Here's the drawing with two shaded views (mm, measured from the low corner). I have some questions. A direction names the side the tool comes from. Give positions to 0.01 mm unless a question says otherwise; leave off trailing zeros. Loops run counter-clockwise (first coordinate to the right, second up) from the corner with the lowest first, then second, coordinate; pieces in that order, holes last. Notation, with made-up numbers: M 4,33.5 L 30,33.5 A26 cw 30,52.5 Z; hole C -34,10 d8. An arc over 180 degrees is marked long. Use a Markdown table: item, result. Add a question column.
1) Suppose I cut it at D-D on x = 24. List the corners of the cut face in (y, z) for me, and give its area (3 significant figures).
2) Suppose I cut it at B-B on x = 42. List the corners of the cut face in (y, z) for me.
3) Suppose I cut it at C-C on z = 42.5. List the corners of the cut face in (x, y) for me.
4) Suppose I cut it at A-A on y = 33.5. List the corners of the cut face in (x, z) for me.
5) We'd pull the mould along Z, two halves only. Please class the marked faces 1, 2 and 3: +Z half, -Z half, draft (parallel to the pull), parting line (faces both ways), or undercut.
6) If I drill on line 1 along Z through (x, y) = (42, 12); line 2 along Z through (x, y) = (9, 33.5); line 3 along X through (y, z) = (28, 15), over which ranges is the centre line in solid material (lowest first)? Write a range as [from, to].
7) Will these pins go through, and if not, where does the flat tip stop? pin 1 Ø12 at (x, z) = (42, 23) entering from -Y; pin 2 Ø1 at (x, z) = (45, 5.5) entering from +Y; pin 3 Ø10 at (y, z) = (17, 22.5) entering from -X; pin 4 Ø8 at (x, z) = (19.5, 19) entering from -Y.
8) Which directions (+Z, -Z, +X, -X, +Y, -Y) give clear straight access to the entire face, cutting with the end or side of a thin tool? Please do the marked faces 4, 5, 6 and 7.
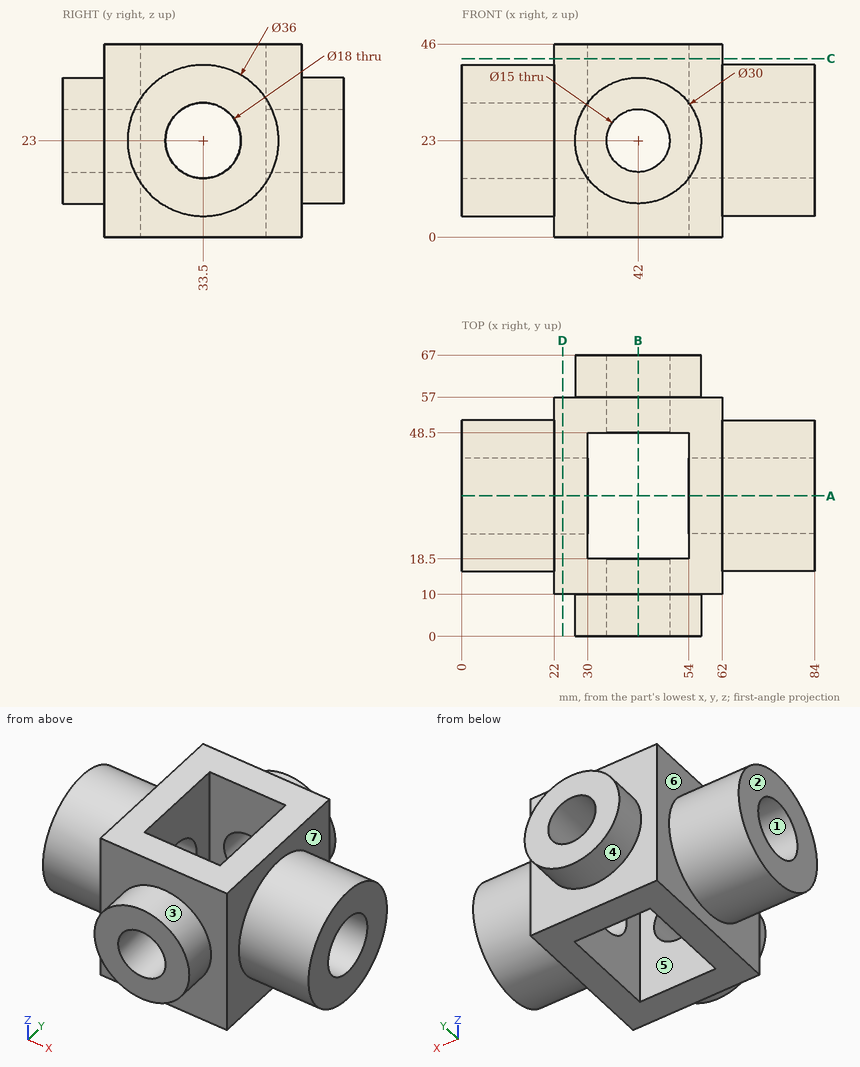
Answer block:
| question | item | result |
|---|---|---|
| 1 | outline | M 10,0 L 57,0 L 57,46 L 10,46 Z; hole C 33.5,23 d18 |
| 1 | area | 1,910 mm^2 |
| 2 | outline | M 0,8 L 10,8 L 10,0 L 18.5,0 L 18.5,15.5 L 0,15.5 Z; M 0,30.5 L 18.5,30.5 L 18.5,46 L 10,46 L 10,38 L 0,38 Z; M 48.5,0 L 57,0 L 57,8 L 67,8 L 67,15.5 L 48.5,15.5 Z; M 48.5,30.5 L 67,30.5 L 67,38 L 57,38 L 57,46 L 48.5,46 Z |
| 3 | outline | M 22,10 L 62,10 L 62,57 L 22,57 Z; hole M 30,18.5 L 54,18.5 L 54,48.5 L 30,48.5 Z |
| 4 | outline | M 0,5 L 22,5 L 22,0 L 30,0 L 30,14 L 0,14 Z; M 0,32 L 30,32 L 30,46 L 22,46 L 22,41 L 0,41 Z; M 54,0 L 62,0 L 62,5 L 84,5 L 84,14 L 54,14 Z; M 54,32 L 84,32 L 84,41 L 62,41 L 62,46 L 54,46 Z |
| 5 | face 1 | undercut |
| 5 | face 2 | draft |
| 5 | face 3 | parting line |
| 6 | line 1 | z = [0, 15.5], [30.5, 46] |
| 6 | line 2 | z = [5, 14], [32, 41] |
| 6 | line 3 | x = [0, 30], [54, 84] |
| 7 | pin 1 | passes through |
| 7 | pin 2 | stops at y = 57 |
| 7 | pin 3 | stops at x = 0 |
| 7 | pin 4 | stops at y = 10 |
| 8 | face 4 | +Y |
| 8 | face 5 | +Z, -Z |
| 8 | face 6 | -X |
| 8 | face 7 | +X |
